Autodesk Inventor part; units mm, degrees
ref_plane "YZ Plane" through (0, 0, 0) normal (1, 0, 0) x (0, 1, 0)
ref_plane "XZ Plane" through (0, 0, 0) normal (0, 1, 0) x (-1, 0, 0)
ref_plane "XY Plane" through (0, 0, 0) normal (0, 0, 1) x (1, 0, 0)
sketch "Sketch1" plane through (0, 0, 0) normal (0, 0, 1) x (1, 0, 0)
  line L0 (-50, 0) -> (-47, 0)
  line L1 (-47, 0) -> (-47, -25)
  line L2 (-47, -25) -> (-48, -25)
  line L3 (-50, -23) -> (-50, 0)
  line L4 (-47, 20) -> (-50, 20)
  line L5 (-50, 20) -> (-50, 58)
  line L6 (-48, 60) -> (-47, 60)
  line L7 (-47, 60) -> (-47, 20)
  line L8 (-50, 0) -> (-65, 0)
  line L9 (-65, 0) -> (-50, 20)
  line L10 (-47, 20) -> (-47, 0)
  arc A0 (-48, 60) -> (-50, 58) centre (-48, 58) ccw
  arc A1 (-50, -23) -> (-48, -25) centre (-48, -23) ccw
  line L11 (0, -42.5799) -> (0, 77.5799)
  point P0 (0, 0)
  point P1 (-50, -25)
  point P2 (-50, 60)
  point P3 (-48.5, 0)
  dimension "d4" = 3
  dimension "d5" = 25
  dimension "d6" = 3
  dimension "d7" = 40
  dimension "d8" = 15
  dimension "d9" = 50
  dimension "d10" = 2
  dimension "d12" = 20
revolve "Revolution1" add sketch "Sketch1" angle 360 about axis through (0, -10, 0) along (0, 1, 0)
sketch "Sketch2" plane through (0, -25, 0) normal (0, -1, 0) x (1, 0, 0)
  line L0 (1.5, 42) -> (-1.5, 42)
  line L1 (-1.5, 42) -> (-1.5, 52)
  line L2 (-1.5, 52) -> (1.5, 52)
  line L3 (1.5, 52) -> (1.5, 42)
  circle A0 centre (0, 0) radius 47
  line L4 (1.5, 42) -> (-1.5, 52) construction
  line L5 (-1.5, 42) -> (1.5, 52) construction
  point P0 (0, 47)
  dimension "d13" = 3
  dimension "d14" = 10
extrude "Extrusion1" cut sketch "Sketch2" against normal blind 25 contours L0 L1 A0 L3 | A0 L1 L2 L3 picked at (0.1667, 43.6658)
pattern_circular "Circular Pattern1" count 6 over 360 about axis through (0, -10, 0) along (0, 1, 0) of "Extrusion1"
properties part number "top-ventilation-tibe-adapter-100mmID-to-100mmID"
Geometry check sheet. Reference: the model listing, model coordinates, mm. A direction names the side the tool comes from. Give positions to 0.01 mm unless a question says otherwise; leave off trailing zeros. Loops run counter-clockwise (first coordinate to the right, second up) from the corner with the lowest first, then second, coordinate; pieces in that order, holes last.
(1) Thickness scan on L1, parallel to X at y = 44, z = -1; L2, parallel to Z at x = 0, y = 4; L3, parallel to Z at x = -11, y = 1.5. Record the ranges inside material, lowest first.
From the geometry:
L1: x = -49.99 to -46.99, 46.99 to 49.99
L2: z = -62 to -47, 47 to 62
L3: z = -62.92 to -45.69, 45.69 to 62.92
(2) Depth check by flat-ended pin: pin 1 Ø1 at (x, y) = (-9, 34.5) entering from +Z; pin 2 Ø5 at (y, z) = (47.5, 12) entering from +X; pin 3 Ø4 at (y, z) = (46.5, 32) entering from -X. Enter the tip coordinate at first touch or a pass-through.
From the geometry:
pin 1: stops at z = 49.27
pin 2: stops at x = 49.09
pin 3: stops at x = -40
(3) Section check B-B on y = -16. Record the cut outline in (x, z).
From the geometry:
outline: (-44.03, -23.69) - (-41.43, -22.19) arc R47 cw to (-41.43, 22.19) - (-44.03, 23.69) arc R50 ccw to start; (-42.53, -26.29) arc R50 ccw to (-1.5, -49.98) - (-1.5, -46.98) arc R47 cw to (-39.93, -24.79) - close; (-42.53, 26.29) - (-39.93, 24.79) arc R47 cw to (-1.5, 46.98) - (-1.5, 49.98) arc R50 ccw to start; (1.5, -49.98) arc R50 ccw to (42.53, -26.29) - (39.93, -24.79) arc R47 cw to (1.5, -46.98) - close; (1.5, 46.98) arc R47 cw to (39.93, 24.79) - (42.53, 26.29) arc R50 ccw to (1.5, 49.98) - close; (41.43, -22.19) - (44.03, -23.69) arc R50 ccw to (44.03, 23.69) - (41.43, 22.19) arc R47 cw to start
(4) Set-up check for faces 1 (the cylindrical face through (24.7, -11.339, 43.473)), 2 (the cylindrical face through (-50, -11, 0)), 3 (the cylindrical face through (50, -11, 0)), 4 (the cylindrical face through (-24.7, -11.339, -43.473)), 5 (the cylindrical face through (-47.69, 39.27, 15.02)): record each of +Z, -Z, +X, -X, +Y, -Y from which the full face is reachable in a straight line by a thin tool's end or side.
From the geometry:
face 1: +Z, +X, -Y
face 2: -X, -Y
face 3: +X, -Y
face 4: -Z, -X, -Y
face 5: +Y
(5) Section check C-C on y = 44. Record the cut outline in (x, z).
From the geometry:
outline: circle Ø100 at (0, 0); hole circle Ø94 at (0, 0)
(6) Section check A-A on z = 0. Record the cut outline in (x, y).
From the geometry:
outline: (-65, 0) - (-50, 0) - (-50, -23) arc R2 ccw to (-48, -25) - (-47, -25) - (-47, 60) - (-48, 60) arc R2 ccw to (-50, 58) - (-50, 20) - close; (47, -25) - (48, -25) arc R2 ccw to (50, -23) - (50, 0) - (65, 0) - (50, 20) - (50, 58) arc R2 ccw to (48, 60) - (47, 60) - close
(7) Release check for a two-part mould opening along X. For faces 6 (the cylindrical face through (-44.83, 16.9, -14.12)), 7 (the cylindrical face through (25.299, -11.339, -43.127)), 8 (the cylindrical face through (-25.299, -11.339, 43.127)), 9 (the flat face through (-24, -25, 41)) record: released by +X, released by -X, zero draft, split by the parting line, or undercut.
From the geometry:
face 6: undercut
face 7: released by +X
face 8: released by -X
face 9: zero draft
